The figure shows three views and two pictorial views of one solid part (mm, origin at its lowest corner). Answer the questions. A direction names the side the tool comes from. Coordinates: 2 decimals unless noted, no trailing zeros. Write each loop counter-clockwise with the first axis right and the second up, starting at its lowest first coordinate (ties: lowest second). Pieces come first, ordered by that corner, then holes.
Item 1: Determine the mould class of the marked faces 1, 2 and 3 for opening direction X: released by +X, released by -X, zero draft, split by the parting line, or undercut.
Item 2: Section B-B (z = 6.5) is taken. Give the vertices of the cut face in (x, y), then the cut area to 4 significant figures.
Item 3: Section A-A (x = 26) is taken. Give the vertices of the cut face in (y, z), then the cut area to 3 significant figures.
Item 4: A tool of negligible diameter and unlimited length cuts with its end or side. For the marked faces 4, 5 and 6, from which of +Z, -Z, +X, -X, +Y, -Y can it reach the whole face along a straight path? Write none if from no direction.
Item 5: Section C-C (y = 16.5) is taken. Give the vertices of the cut face in (x, z).
Item 6: Straight lines are drawn through the part: probe 1 along X at (y, z) = (8.25, 5); probe 2 along X at (y, z) = (18.5, 1.5); probe 3 along Y at (x, z) = (36, 1.5). For each, find the intervals that lie inside material, in ascending order.
Item 7: Section D-D (z = 8.5) is taken. Give the vertices of the cut face in (x, y), then the cut area to 3 significant figures.
Item 8: Each of these flat-tipped pins is pushed along its axis until it touches: P1, Ø10, axis at x = 7.5, y = 9, coming from the -Z side; P2, Ø1.2, axis at x = 16.5, z = 1.5, coming from the +Y side. Where does it stop, or does it pass through?
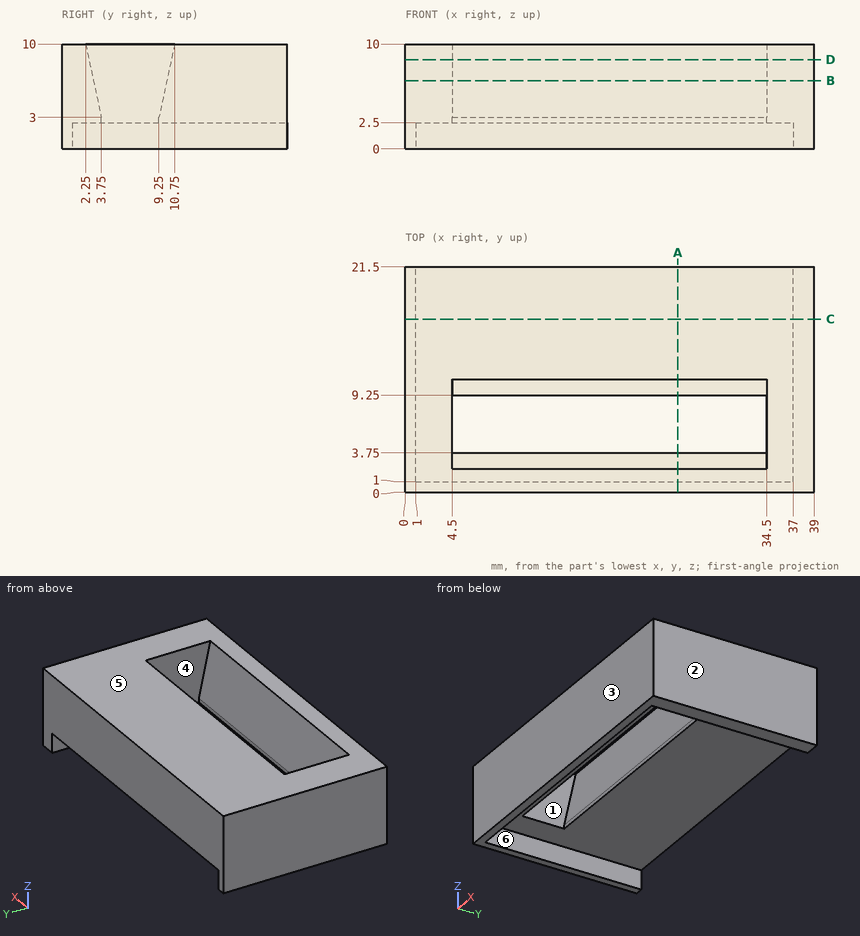
Established:
1. face 1: undercut
1. face 2: released by +X
1. face 3: zero draft
2. outline: (0, 0) - (39, 0) - (39, 21.5) - (0, 21.5) - close; hole (4.5, 3) - (34.5, 3) - (34.5, 10) - (4.5, 10) - close
2. area: 628.5 mm2
3. outline: (0, 0) - (1, 0) - (1, 2.5) - (3.75, 2.5) - (3.75, 3) - (2.25, 10) - (0, 10) - close; (9.25, 2.5) - (21.5, 2.5) - (21.5, 10) - (10.75, 10) - (9.25, 3) - close
3. area: 112 mm2
4. face 4: +Z
4. face 5: +Z, +X, -X, +Y, -Y
4. face 6: -Z, +Y
5. outline: (0, 0) - (1, 0) - (1, 2.5) - (37, 2.5) - (37, 0) - (39, 0) - (39, 10) - (0, 10) - close
6. probe 1: x = 0 to 4.5, 34.5 to 39
6. probe 2: x = 0 to 1, 37 to 39
6. probe 3: y = 0 to 1
7. outline: (0, 0) - (39, 0) - (39, 21.5) - (0, 21.5) - close; hole (4.5, 2.57) - (34.5, 2.57) - (34.5, 10.43) - (4.5, 10.43) - close
7. area: 603 mm2
8. P1: stops at z = 2.5
8. P2: stops at y = 1
